Autodesk Fusion 360 part; units mm, degrees
sketch "Sketch1" plane through (0, 0, 0) normal (0, 0, 1) x (1, 0, 0)
  line L0 (0, 0) -> (-25, 0) construction
  line L1 (0, 0) -> (25, 0) construction
  line L2 (25, 0) -> (25, 10)
  line L3 (25, 0) -> (25, -10)
  line L4 (25, 10) -> (-25, 10)
  line L5 (-25, 10) -> (-25, 0)
  line L6 (-25, 0) -> (-25, -10)
  line L7 (-25, -10) -> (25, -10)
  line L8 (25, 10) -> (40, 10)
  line L9 (40, 10) -> (40, -10)
  line L10 (40, -10) -> (25, -10)
  line L11 (-25, 10) -> (-40, 10)
  line L12 (-40, 10) -> (-40, -10)
  line L13 (-40, -10) -> (-25, -10)
  line L14 (-40, -10) -> (-25, 10) construction
  line L15 (-40, 10) -> (-25, -10) construction
  line L16 (25, -10) -> (40, 10) construction
  line L17 (25, 10) -> (40, -10) construction
  circle A0 centre (-32.5, 0) radius 1.5
  circle A1 centre (-32.5, 0) radius 4.5
  circle A2 centre (32.5, 0) radius 1.5
  circle A3 centre (32.5, 0) radius 4.5
  dimension "d6" = 20
  dimension "d7" = 50
  dimension "d8" = 15
  dimension "d9" = 15
  dimension "d10" = 3
  dimension "d11" = 9
  dimension "d12" = 3
  dimension "d13" = 9
extrude "Extrude3" add sketch "Sketch1" along normal blind 5 contours L2 L3 L4 L5 L6 L7
extrude "Extrude2" add sketch "Sketch1" along normal blind 5 contours L2 L3 L4 L5 L6 L7 | L2 L3 L8 L9 L10 | L5 L6 L11 L12 L13
extrude "Extrude1" add sketch "Sketch1" along normal blind 3 contours L2 L3 L4 L5 L6 L7 | L2 L3 L8 L9 L10 | L5 L6 L11 L12 L13 | A1 | A3
chamfer "Chamfer4" distance 1 angle 45 2 edges at (-33.8985, 0.5424, 3) (31.1015, 0.5424, 3)
fillet "Fillet1" radius 5 4 edges at (40, 10, 2.5) (-40, 10, 2.5) (-40, -10, 2.5) (40, -10, 2.5)
sketch "Sketch2" plane through (0, 0, 5) normal (0, 0, 1) x (-1, 0, 0)
  line L0 (35, 10) -> (-35, 10)
  line L1 (-35, -10) -> (35, -10)
  line L2 (19.6294, -5) -> (-19.6294, -5)
  line L3 (-19.6294, -5) -> (-19.6294, 5)
  line L4 (-19.6294, 5) -> (19.6294, 5)
  line L5 (19.6294, 5) -> (19.6294, -5)
  line L6 (-25, -10) -> (25, -10)
  line L7 (25, 10) -> (-25, 10)
  circle A0 centre (32.5, 0) radius 4.5
  circle A1 centre (-32.5, 0) radius 4.5
  arc A2 (40, 5) -> (35, 10) centre (35, 5) ccw
  line L8 (-40, 5) -> (-40, -5)
  arc A3 (-40, -5) -> (-35, -10) centre (-35, -5) ccw
  arc A4 (35, -10) -> (40, -5) centre (35, -5) ccw
  line L9 (40, -5) -> (40, 5)
  arc A5 (-35, 10) -> (-40, 5) centre (-35, 5) ccw
  dimension "d26" = 5
  dimension "d27" = 5
extrude "Extrude4" add sketch "Sketch2" along normal blind 30 contours L2 L3 L4 L5
fillet "Fillet4" radius 3.5 4 edges at (19.6294, 0, 5) (-19.6294, 0, 5) (0, 5, 5) (0, -5, 5)
fillet "Fillet5" radius 3 2 edges at (-19.6294, 0, 35) (19.6294, 0, 35)
sketch "Sketch3" plane through (0, 5, 0) normal (0, 1, 0) x (-1, 0, 0)
  line L0 (-19.6294, 8.5) -> (19.6294, 8.5)
  line L1 (19.6294, 8.5) -> (19.6294, 32)
  line L2 (16.6294, 35) -> (-16.6294, 35)
  line L3 (-19.6294, 32) -> (-19.6294, 8.5)
  line L4 (0, 35) -> (0, 0) construction
  line L5 (-17.1147, 29.85) -> (-2.5147, 29.85)
  line L6 (-2.5147, 29.85) -> (-2.5147, 13.65)
  line L7 (-2.5147, 13.65) -> (-17.1147, 13.65)
  line L8 (-17.1147, 13.65) -> (-17.1147, 29.85)
  line L9 (2.5147, 29.85) -> (17.1147, 29.85)
  line L10 (17.1147, 29.85) -> (17.1147, 13.65)
  line L11 (17.1147, 13.65) -> (2.5147, 13.65)
  line L12 (2.5147, 13.65) -> (2.5147, 29.85)
  line L13 (-2.5147, 29.85) -> (0, 29.85) construction
  line L14 (-17.1147, 29.85) -> (-19.6294, 29.85) construction
  line L15 (-2.5147, 29.85) -> (-2.5147, 35) construction
  line L16 (-17.1147, 13.65) -> (-17.1147, 8.5) construction
  line L17 (2.5147, 29.85) -> (2.5147, 35) construction
  line L18 (17.1147, 13.65) -> (17.1147, 8.5) construction
  line L19 (0, 29.85) -> (2.5147, 29.85) construction
  line L20 (17.1147, 13.65) -> (19.6294, 13.65) construction
  arc A0 (-16.6294, 35) -> (-19.6294, 32) centre (-16.6294, 32) ccw
  arc A1 (19.6294, 32) -> (16.6294, 35) centre (16.6294, 32) ccw
  dimension "d31" = 14.6
  dimension "d32" = 16.2
extrude "Extrude5" cut sketch "Sketch3" against normal blind 10 contours L5 L6 L7 L8 | L9 L10 L11 L12
sketch "Sketch4" plane through (0, 5, 0) normal (0, 1, 0) x (-1, 0, 0)
  line L0 (-2.5147, 29.85) -> (-2.5147, 13.65)
  line L1 (-2.5147, 13.65) -> (-17.1147, 13.65)
  line L2 (-17.1147, 13.65) -> (-17.1147, 29.85)
  line L3 (-17.1147, 29.85) -> (-2.5147, 29.85)
  line L4 (17.1147, 29.85) -> (17.1147, 13.65)
  line L5 (17.1147, 13.65) -> (2.5147, 13.65)
  line L6 (2.5147, 13.65) -> (2.5147, 29.85)
  line L7 (2.5147, 29.85) -> (17.1147, 29.85)
  arc A0 (-16.6294, 35) -> (-19.6294, 32) centre (-16.6294, 32) ccw
  line L8 (-19.6294, 32) -> (-19.6294, 8.5)
  line L9 (-19.6294, 8.5) -> (19.6294, 8.5)
  line L10 (19.6294, 8.5) -> (19.6294, 32)
  arc A1 (19.6294, 32) -> (16.6294, 35) centre (16.6294, 32) ccw
  line L11 (16.6294, 35) -> (-16.6294, 35)
  line L12 (-2.5147, 29.85) -> (-2.5147, 13.65)
  line L13 (-17.1147, 29.85) -> (-2.5147, 29.85)
  line L14 (-17.1147, 13.65) -> (-17.1147, 29.85)
  line L15 (-2.5147, 13.65) -> (-17.1147, 13.65)
  line L16 (17.1147, 29.85) -> (17.1147, 13.65)
  line L17 (17.1147, 13.65) -> (2.5147, 13.65)
  line L18 (2.5147, 13.65) -> (2.5147, 29.85)
  line L19 (2.5147, 29.85) -> (17.1147, 29.85)
  line L20 (-17.2147, 31.35) -> (-2.4147, 31.35)
  line L21 (-2.4147, 31.35) -> (-2.4147, 9.65)
  line L22 (-2.4147, 9.65) -> (-17.2147, 9.65)
  line L23 (-17.2147, 9.65) -> (-17.2147, 31.35)
  line L24 (2.4147, 31.35) -> (17.2147, 31.35)
  line L25 (17.2147, 31.35) -> (17.2147, 9.65)
  line L26 (17.2147, 9.65) -> (2.4147, 9.65)
  line L27 (2.4147, 9.65) -> (2.4147, 31.35)
  dimension "d38" = 4
  dimension "d39" = 0.1
  dimension "d40" = 0.1
  dimension "d41" = 1.5
  dimension "d42" = 0.1
  dimension "d43" = 0.1
  dimension "d44" = 4
  dimension "d45" = 1.5
extrude "Extrude6" cut sketch "Sketch4" against normal blind 8 contours L20 L21 L22 L23 | L24 L25 L26 L27
sketch "Sketch5" plane through (0, 0, 9.65) normal (0, 0, 1) x (-1, 0, 0)
  line L0 (-17.2147, -5) -> (-2.4147, -5)
  line L1 (-2.4147, -5) -> (-2.4147, 3)
  line L2 (-2.4147, 3) -> (-17.2147, 3)
  line L3 (-17.2147, 3) -> (-17.2147, -5)
  line L4 (-17.1147, 3) -> (-2.5147, 3)
  line L5 (-2.5147, 3) -> (-2.5147, 5)
  line L6 (-2.5147, 5) -> (-17.1147, 5)
  line L7 (-17.1147, 5) -> (-17.1147, 3)
  line L8 (2.4147, -5) -> (17.2147, -5)
  line L9 (17.2147, -5) -> (17.2147, 3)
  line L10 (17.2147, 3) -> (2.4147, 3)
  line L11 (2.4147, 3) -> (2.4147, -5)
  line L12 (2.5147, 3) -> (17.1147, 3)
  line L13 (17.1147, 3) -> (17.1147, 5)
  line L14 (17.1147, 5) -> (2.5147, 5)
  line L15 (2.5147, 5) -> (2.5147, 3)
  line L16 (2.4147, -3.25) -> (17.2147, -3.25)
  line L17 (-2.4147, -3.25) -> (-17.2147, -3.25)
  dimension "d49" = 8.25
  dimension "d50" = 8.25
extrude "Extrude7" add sketch "Sketch5" along normal blind 0.5 contours L0 L1 L3 L17 | L8 L9 L11 L16
sketch "Sketch6" plane through (0, 0, 31.35) normal (0, 0, -1) x (1, 0, 0)
  line L0 (2.4147, -5) -> (17.2147, -5)
  line L1 (17.2147, -5) -> (17.2147, 3)
  line L2 (17.2147, 3) -> (2.4147, 3)
  line L3 (2.4147, 3) -> (2.4147, -5)
  line L4 (-2.4147, -5) -> (-17.2147, -5)
  line L5 (-17.2147, -5) -> (-17.2147, -3.25)
  line L6 (-17.2147, -3.25) -> (-2.4147, -3.25)
  line L7 (-2.4147, -3.25) -> (-2.4147, -5)
  line L8 (2.4147, -3.25) -> (17.2147, -3.25)
  line L9 (17.2147, -3.25) -> (17.2147, -5)
  line L10 (17.2147, -5) -> (2.4147, -5)
  line L11 (2.4147, -5) -> (2.4147, -3.25)
extrude "Extrude8" add sketch "Sketch6" along normal blind 0.5 contours L0 L1 L3 L8 L9 L10 L11 | L4 L5 L6 L7
chamfer "Chamfer2" distance 2 angle 55 2 edges at (9.8147, -3, 13.65) (-9.8147, -3, 13.65) measured on face at (7.3814, -3.6667, 13.65) measured on face at (-12.2481, -3.6667, 13.65)
chamfer "Chamfer3" distance 1.5 angle 45 8 edges at (40, 0, 0) (38.5355, 8.5355, 0) (0, 10, 0) (-38.5355, 8.5355, 0) (-40, 0, 0) (-38.5355, -8.5355, 0) (0, -10, 0) (38.5355, -8.5355, 0)
Can you work these out from the model? Positions are in its coordinate system, mm. A direction names the side the tool comes from. Give positions to 0.01 mm unless a question says otherwise; leave off trailing zeros. Write each loop counter-clockwise with the first axis right and the second up, starting at its lowest first coordinate (ties: lowest second). Pieces come first, ordered by that corner, then holes. Notation, with made-up numbers: (0.5, 4) - (44.5, 4) arc R34 ccw to (44.5, 38) - close; hole circle Ø1 at (73.25, -11.5). An arc over 180 degrees is marked (long way). Write item = value, one per line. Start each with the question number.
1. Imagine slicing it at A-A (z = 22). Please give me the cut outline in (x, y), and give its area (3 significant figures).
2. Thinking about a two-plate mould opening in Y: for faces 6 (the face through (10, 0, 31.35)), 7 (the face through (-39, 8, 3)), 8 (the face through (-2.515, -4, 20)), which applies, released by +Y, released by -Y, zero draft, split by the parting line, or undercut?
3. Imagine slicing it at C-C (y = 0). Count the separate pieces of the cut face and the enclosed holes in it, and give its area (3 significant figures).
4. Imagine slicing it at D-D (z = 12.5). Please give me the cut outline in (x, y).
5. For pin 1 (2 mm diameter, centred on y = -3.5, z = 17, fed in from +X); pin 2 (16.5 mm diameter, centred on x = 12, z = 17, fed in from +Y); pin 3 (1.5 mm diameter, centred on y = 0.5, z = 6.5, fed in from -X), each with a flat end and sliding along its axis, tell me the tip position at first contact or that it passes through.
6. Please list where these lines run through material, in increasing order: line 1 (X direction, y = -2.25, z = 26); line 2 (Y direction, x = -32.5, z = 3.6); line 3 (X direction, y = -4, z = 25.5).
7. On a 3-axis mill with a long thin cutter (end or side, diameter ignored), from which of +Z, -Z, +X, -X, +Y, -Y can I reach the whole of each face in a straight line? I mean faces 1 (the face through (-9.8, -3, 30.2)), 2 (the face through (-37.9, -7.9, 0.6)), 3 (the face through (39.2, -0.1, 0.7)), 4 (the face through (-10, 4, 30.85)), 5 (the face through (-1, 9, 5)). Say none if no direction works.
Worked answers:
q1.outline = (-19.63, -5) - (-17.11, -5) - (-17.11, -3) - (-17.21, -3) - (-17.21, 5) - (-19.63, 5) - close; (-2.51, -5) - (2.51, -5) - (2.51, -3) - (2.41, -3) - (2.41, 5) - (-2.41, 5) - (-2.41, -3) - (-2.51, -3) - close; (17.11, -5) - (19.63, -5) - (19.63, 5) - (17.21, 5) - (17.21, -3) - (17.11, -3) - close
q1.area = 97.4 mm2
q2.face_6 = undercut
q2.face_7 = released by +Y
q2.face_8 = zero draft
q3.separate_pieces = 3
q3.enclosed_holes = 2
q3.area = 879 mm2
q4.outline = (-19.63, -5) - (19.63, -5) - (19.63, 5) - (17.21, 5) - (17.21, -3) - (17.11, -3) - (17.11, -4.19) - (2.51, -4.19) - (2.51, -3) - (2.41, -3) - (2.41, 5) - (-2.41, 5) - (-2.41, -3) - (-2.51, -3) - (-2.51, -4.19) - (-17.11, -4.19) - (-17.11, -3) - (-17.21, -3) - (-17.21, 5) - (-19.63, 5) - close
q5.pin_1 = 19.63
q5.pin_2 = 5
q5.pin_3 = -20.96
q6.line_1 = -19.63 to -17.21, -2.41 to 2.41, 17.21 to 19.63
q6.line_2 = -10 to -4.5, 4.5 to 10
q6.line_3 = -19.63 to -17.11, -2.51 to 2.51, 17.11 to 19.63
q7.face_1 = none
q7.face_2 = -Z, -X, -Y
q7.face_3 = -Z, +X, +Y, -Y
q7.face_4 = +Y
q7.face_5 = +Z
